Work out the finished part from the listing and answer in its coordinate system (mm). Face numbers are marked on the shaded views. Round coordinates to 2 decimals unless told otherwise and drop trailing zeros. Write each loop counter-clockwise with the first axis right and the second up, starting at its lowest first coordinate (ties: lowest second). Pieces come first, ordered by that corner, then holes. Notation, with made-up numbers: (46, -35) -> (80, -35) arc R27 ccw to (80, 0) -> close; hole circle Ø10 at (-31, 13.5). An arc over 180 degrees is marked (long way). One line per question, with ' | ' between items. Start each with the question number.
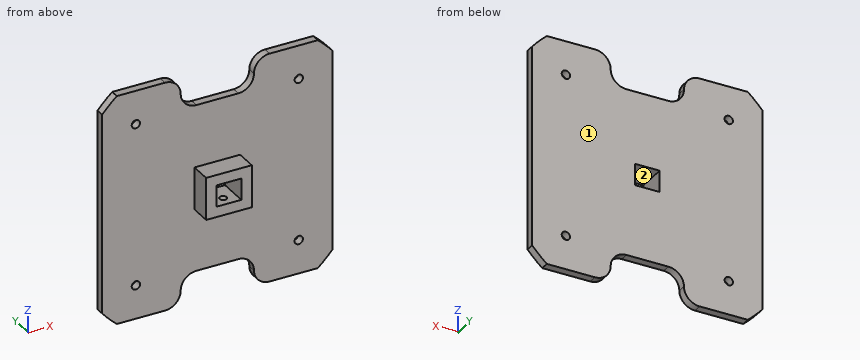
```python
from build123d import *

# Parameters (mm, degrees)
BOSS_EXTRUDE1_DEPTH      = 4
F_4_0MM_DOWEL_HOLE2_D    = 4
FILLET1_START            = -1
FILLET1_DEPTH            = 6
FILLET1_2_DEPTH          = 4
SKETCH7_W                = 21.8
SKETCH7_H                = 20.3
SKETCH7_W_2              = 11.8
SKETCH7_H_2              = 10.3
BOSS_EXTRUDE2_DEPTH      = 10
M3_CLEARANCE_HOLE1_D     = 3.4
M3_CLEARANCE_HOLE1_DEPTH = 5
SKETCH7_2_W              = 11.8
SKETCH7_2_H              = 10.3
CUT_EXTRUDE1_DEPTH       = 10


with BuildPart() as part:
    # Sketch1 → Boss-Extrude1 (new body)
    with BuildSketch(Plane(origin=(0, 0, 0), x_dir=(1, 0, 0), z_dir=(0, 1, 0))):
        with BuildLine():
            Line((55, 48), (55, -48))
            ThreePointArc((55, -48), (51.618795027, -51.618795027), (48, -55))
            Line((48, -55), (17.5, -55))
            Line((17.5, -55), (17.5, -40))
            Line((17.5, -40), (-17.5, -40))
            Line((-17.5, -40), (-17.5, -55))
            Line((-17.5, -55), (-48, -55))
            ThreePointArc((-48, -55), (-51.618795027, -51.618795027), (-55, -48))
            Line((-55, -48), (-55, 48))
            ThreePointArc((-55, 48), (-51.618795027, 51.618795027), (-48, 55))
            Line((-48, 55), (-17.5, 55))
            Line((-17.5, 55), (-17.5, 40))
            Line((-17.5, 40), (17.5, 40))
            Line((17.5, 40), (17.5, 55))
            Line((17.5, 55), (48, 55))
            ThreePointArc((48, 55), (51.618795027, 51.618795027), (55, 48))
        make_face()
    extrude(amount=BOSS_EXTRUDE1_DEPTH)

    # Ø4.0mm Dowel Hole2 (through all)
    with Locations(Plane(origin=(0, 4, 0), x_dir=(1, 0, 0), z_dir=(0, 1, 0))):
        with Locations((38.890872965, 38.890872965), (38.890872965, -38.890872965), (-38.890872965, -38.890872965), (-38.890872965, 38.890872965)):
            Hole(F_4_0MM_DOWEL_HOLE2_D / 2)

    # Fillet1: read off the stored shape, not the designer's step
    # Fillet1 outline → Fillet1 (cut)
    with BuildSketch(Plane(origin=(0, 0, 0), x_dir=(1, 0, 0), z_dir=(0, 1, 0)).offset(FILLET1_START)):
        with BuildLine():
            Line((17.5, 55), (17.5, 47.5))
            ThreePointArc((17.5, 47.5), (19.696699141, 52.803300859), (25, 55))
            Line((25, 55), (17.5, 55))
        make_face()
        with BuildLine():
            ThreePointArc((-25, 55), (-19.696699141, 52.803300859), (-17.5, 47.5))
            Line((-17.5, 47.5), (-17.5, 55))
            Line((-17.5, 55), (-25, 55))
        make_face()
        with BuildLine():
            Line((-17.5, -55), (-17.5, -47.5))
            ThreePointArc((-17.5, -47.5), (-19.696699141, -52.803300859), (-25, -55))
            Line((-25, -55), (-17.5, -55))
        make_face()
        with BuildLine():
            ThreePointArc((25, -55), (19.696699141, -52.803300859), (17.5, -47.5))
            Line((17.5, -47.5), (17.5, -55))
            Line((17.5, -55), (25, -55))
        make_face()
    extrude(amount=FILLET1_DEPTH, mode=Mode.SUBTRACT)

    # Fillet1 2 outline → Fillet1 2 (add)
    with BuildSketch(Plane(origin=(0, 0, 0), x_dir=(1, 0, 0), z_dir=(0, 1, 0))):
        with BuildLine():
            Line((-17.5, 40), (-10, 40))
            ThreePointArc((-10, 40), (-15.303300859, 42.196699141), (-17.5, 47.5))
            Line((-17.5, 47.5), (-17.5, 40))
        make_face()
        with BuildLine():
            ThreePointArc((17.5, 47.5), (15.303300859, 42.196699141), (10, 40))
            Line((10, 40), (17.5, 40))
            Line((17.5, 40), (17.5, 47.5))
        make_face()
        with BuildLine():
            Line((17.5, -40), (10, -40))
            ThreePointArc((10, -40), (15.303300859, -42.196699141), (17.5, -47.5))
            Line((17.5, -47.5), (17.5, -40))
        make_face()
        with BuildLine():
            ThreePointArc((-17.5, -47.5), (-15.303300859, -42.196699141), (-10, -40))
            Line((-10, -40), (-17.5, -40))
            Line((-17.5, -40), (-17.5, -47.5))
        make_face()
    extrude(amount=FILLET1_2_DEPTH)

    # Sketch7 → Boss-Extrude2 (add)
    with BuildSketch(Plane.XZ):
        Rectangle(SKETCH7_W, SKETCH7_H)
        Rectangle(SKETCH7_W_2, SKETCH7_H_2, mode=Mode.SUBTRACT)
    extrude(amount=BOSS_EXTRUDE2_DEPTH)

    # M3 Clearance Hole1
    with Locations(Plane(origin=(0, -5, -10.15), x_dir=(-1, 0, 0), z_dir=(0, 0, -1))):
        with Locations((0, 0)):
            Hole(M3_CLEARANCE_HOLE1_D / 2, depth=M3_CLEARANCE_HOLE1_DEPTH)

    # Sketch7<2> → Cut-Extrude1 (cut)
    with BuildSketch(Plane.XZ):
        Rectangle(SKETCH7_2_W, SKETCH7_2_H)
    extrude(amount=-CUT_EXTRUDE1_DEPTH, mode=Mode.SUBTRACT)


solid = part.part
```
(1) A cutting plane is placed at C-C, the plane z = -13. Determine the outline of the cut face in (x, y), then the cut area to 3 significant figures.
(2) A cutting plane is placed at B-B, the plane x = 0. Determine the outline of the cut face in (y, z).
(3) The mould has two halves that part along X. Classify the marked faces 1 and 2: +X half, -X half, draft (parallel to the pull), parting line (faces both ways), or undercut.
(4) Given pin 1 Ø4.5 at (x, y) = (0, -5) entering from +Z; pin 2 Ø4.5 at (x, y) = (3, 2) entering from +Z; pin 3 Ø1.5 at (y, z) = (-3.5, 5) entering from -X, each flat-ended and moving along its own axis, determine where each tip first touches the part or whether it passes through.
(5) A cutting plane is placed at A-A, the plane y = -1.25. Determine the outline of the cut face in (x, z).
(6) Consider L1, parallel to X at y = -5, z = -3.5; L2, parallel to Z at x = -40, y = 3.5; L3, parallel to Y at x = -31, z = 35.5. Determine where each line is inside the solid, lowest interval first.
Returned:
1) outline: (-55, 0) -> (55, 0) -> (55, 4) -> (-55, 4) -> close | area: 440 mm2
2) outline: (-10, -10.15) -> (-6.7, -10.15) -> (-6.7, -5.15) -> (-10, -5.15) -> close; (-10, 5.15) -> (4, 5.15) -> (4, 40) -> (0, 40) -> (0, 10.15) -> (-10, 10.15) -> close; (-3.3, -10.15) -> (0, -10.15) -> (0, -40) -> (4, -40) -> (4, -5.15) -> (-3.3, -5.15) -> close
3) face 1: draft | face 2: undercut
4) pin 1: z = 10.15 | pin 2: z = 40 | pin 3: x = -10.9
5) outline: (-10.9, -10.15) -> (10.9, -10.15) -> (10.9, 10.15) -> (-10.9, 10.15) -> close; hole (-5.9, -5.15) -> (5.9, -5.15) -> (5.9, 5.15) -> (-5.9, 5.15) -> close
6) L1: -10.9 to -5.9, 5.9 to 10.9 | L2: -55 to -40.56, -37.23 to 37.23, 40.56 to 55 | L3: 0 to 4
